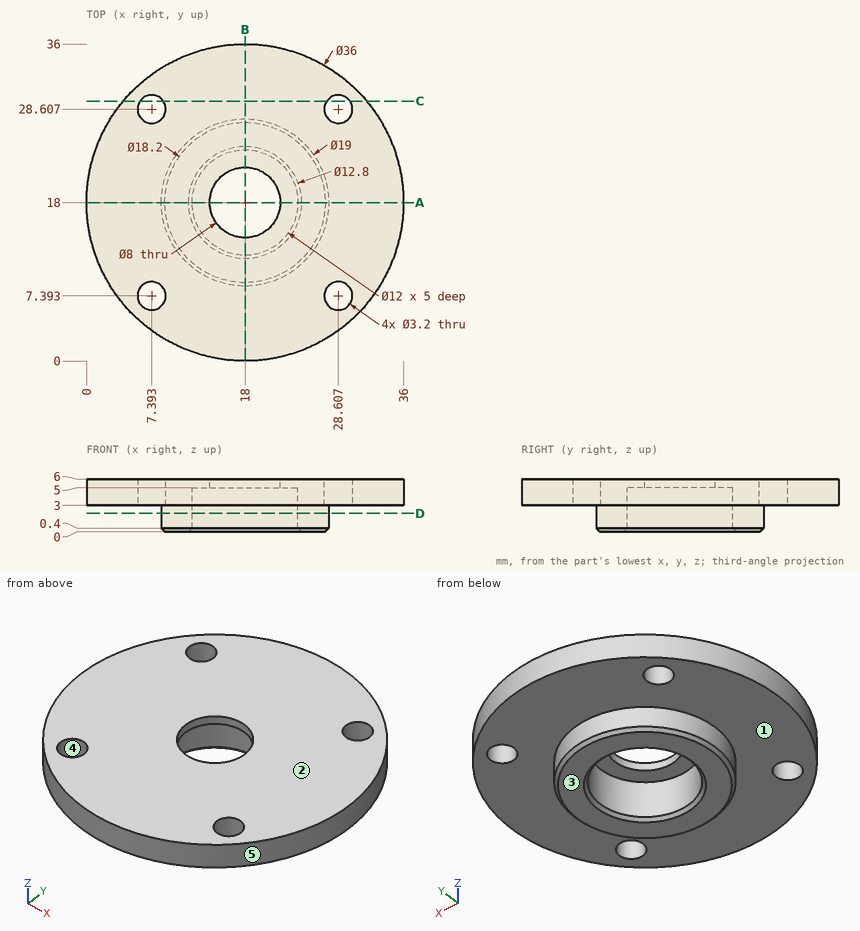
Geometry check sheet. Reference: drawing and pictorial views, mm from the part's lowest x, y, z. A direction names the side the tool comes from. Give positions to 0.01 mm unless a question says otherwise; leave off trailing zeros. Write each loop counter-clockwise with the first axis right and the second up, starting at its lowest first coordinate (ties: lowest second). Pieces come first, ordered by that corner, then holes. Notation, with made-up numbers: M 38.5,6 L 81.5,6 A19 cw 81.5,22 Z; hole C -12,-27.75 d10. An arc over 180 degrees is marked long. Answer as CSV lines item,"result". Start each with the question number.
Q1. Tool access check on the marked faces 1 and 2. Record the directions out of +Z, -Z, +X, -X, +Y, -Y that give a thin tool (end or side, any length) a straight path to the whole face; none if there is none.
Q2. Section check D-D, the plane z = 2.1. Record the cut outline in (x, y).
Q3. Material ranges on L1, parallel to Y at x = 18, z = 2.45; L2, parallel to X at y = 30, z = 3.25 (1 decimal); L3, parallel to Z at x = 7, y = 22, recorded low to high.
Q4. Go/stop test with flat-tipped pins: pin 1 (4 mm diameter, centred on x = 7.39, y = 7.39, fed in from -Z); pin 2 (2 mm diameter, centred on x = 18, z = 3, fed in from -Y); pin 3 (2 mm diameter, centred on y = 16, z = 1, fed in from +X). Record where each tip stops, or that it passes through.
Q5. Section check A-A, the plane y = 18. Record the cut outline in (x, z).
Q6. Section check C-C, the plane y = 29.5. Record the cut outline in (x, z).
Q7. Release check for a two-part mould opening along X. For the marked faces 3, 4 and 5 record: pulls with the +X half, pulls with the -X half, needs draft (parallel to the pull), parting line crosses it, or undercut.
Geometry says:
1,face 1,"-Z"
1,face 2,"+Z, +X, -X, +Y, -Y"
2,outline,"C 18,18 d19; hole C 18,18 d12"
3,L1,"8.5 to 12, 24 to 27.5"
3,L2,"4.6 to 6.6, 8.2 to 27.8, 29.4 to 31.4"
3,L3,"3 to 6"
4,pin 1,"z = 3"
4,pin 2,"y = 0"
4,pin 3,"x = 27.45"
5,outline,"M 0,3 L 8.5,3 L 8.5,0.4 L 8.9,0 L 11.6,0 L 12,0.4 L 12,5 L 14,5 L 14,6 L 0,6 Z; M 22,5 L 24,5 L 24,0.4 L 24.4,0 L 27.1,0 L 27.5,0.4 L 27.5,3 L 36,3 L 36,6 L 22,6 Z"
6,outline,"M 4.15,3 L 6.07,3 L 6.07,6 L 4.15,6 Z; M 8.72,3 L 27.28,3 L 27.28,6 L 8.72,6 Z; M 29.93,3 L 31.85,3 L 31.85,6 L 29.93,6 Z"
7,face 3,"needs draft"
7,face 4,"undercut"
7,face 5,"parting line crosses it"
